```python
from build123d import *

# Parameters (mm, degrees)
SKETCH1_W           = 32
SKETCH1_H           = 32
BOSS_EXTRUDE1_DEPTH = 3.5


with BuildPart() as part:
    # Sketch1 → Boss-Extrude1 (new body, symmetric)
    with BuildSketch(Plane(origin=(0, 0, 0), x_dir=(1, 0, 0), z_dir=(0, 1, 0))):
        Rectangle(SKETCH1_W, SKETCH1_H)
    extrude(amount=BOSS_EXTRUDE1_DEPTH, both=True)

    # Sketch2 → Cut-Revolve1 (revolve, cut)
    with BuildSketch(Plane.XY):
        Polygon((8, 3.5), (14.5, 3.5), (11.613248654, -1.5), (11.613248654, -3.5), (8, -3.5), align=None)
    cut_revolve1 = revolve(axis=Axis((8, 3.5, 0), (0, -1, 0)), mode=Mode.SUBTRACT)

    # Mirror1: Cut-Revolve1 across plane
    add(cut_revolve1.mirror(Plane(origin=(0, 0, 0), x_dir=(0, 0, 1), z_dir=(1, 0, 0))), mode=Mode.SUBTRACT)


solid = part.part
```
For this review, take the finished solid that the model builds, in its own axes (mm). Give positions to 0.01 mm unless a question says otherwise; leave off trailing zeros. Loops run counter-clockwise (first coordinate to the right, second up) from the corner with the lowest first, then second, coordinate; pieces in that order, holes last. Notation, with made-up numbers: M 26,9 L 75,9 A18 ccw 75,18 Z; hole C -36.5,83.5 d5. An arc over 180 degrees is marked long. One line per item, written item: value. Start each with the question number.
Q1. Clearance check with a flat-ended pin moving along its axis: pin 1 Ø9.5 at (x, z) = (-8, 0) entering from +Y. State where the tip first meets the part, or that it passes through.
Q2. Add section B-B (x = 8). Give the boundary of the cut face in (y, z), and give its area (3 significant figures).
Q3. Add section D-D (y = 2.25). Give the boundary of the cut face in (x, z).
Q4. Add section C-C (y = -2.5). Give the boundary of the cut face in (x, z), and give its area (3 significant figures).
Q5. Draft analysis for pull direction Z (two halves, no side actions). For faces 1 (the face through (-4.39, -2.51, 0.16)), 2 (the face through (16, 0, 0)), 3 (the face through (5.02, -1.26, -2.28)), 4 (the face through (0, 0, 16)), state which applies: released by +Z, released by -Z, zero draft, split by the parting line, or undercut.
Q6. For L1, parallel to Z at x = -8, y = -2.75; L2, parallel to X at y = 1.75, z = -2.5; L3, parallel to X at y = -3, z = 3, list the stretches that pass through material, from the lowest coordinate up.
Q7. Add section A-A (z = 0). Give the boundary of the cut face in (x, y).
Reply:
1. pin 1: y = 0.47
2. outline: M -3.5,-16 L 3.5,-16 L 3.5,-6.5 L -1.5,-3.61 L -3.5,-3.61 Z; M -3.5,3.61 L -1.5,3.61 L 3.5,6.5 L 3.5,16 L -3.5,16 Z
2. area: 159 mm²
3. outline: M -16,-16 L 16,-16 L 16,16 L -16,16 Z; hole C -8,0 d11.56; hole C 8,0 d11.56
4. outline: M -16,-16 L 16,-16 L 16,16 L -16,16 Z; hole C -8,0 d7.23; hole C 8,0 d7.23
4. area: 942 mm²
5. face 1: undercut
5. face 2: zero draft
5. face 3: undercut
5. face 4: released by +Z
6. L1: -16 to -3.61, 3.61 to 16
6. L2: -16 to -12.89, -3.11 to 3.11, 12.89 to 16
6. L3: -16 to -10.01, -5.99 to 5.99, 10.01 to 16
7. outline: M -16,-3.5 L -11.61,-3.5 L -11.61,-1.5 L -14.5,3.5 L -16,3.5 Z; M -4.39,-3.5 L 4.39,-3.5 L 4.39,-1.5 L 1.5,3.5 L -1.5,3.5 L -4.39,-1.5 Z; M 11.61,-3.5 L 16,-3.5 L 16,3.5 L 14.5,3.5 L 11.61,-1.5 Z
